Build history of the part. All positions in model axes, mm. Round coordinates to 2 decimals unless told otherwise and drop trailing zeros. Write each loop counter-clockwise with the first axis right and the second up, starting at its lowest first coordinate (ties: lowest second). Pieces come first, ordered by that corner, then holes.
1) Pull direction X, two halves, no side cores. Call faces 1 (the flat face through (0, 6, 5)), 2 (the cylindrical face through (9, -9, 5)), 3 (the flat face through (7, 6, 10)), 4 (the cylindrical face through (6.47, 10.31, 4.93)): +X half, -X half, draft (parallel to the pull), parting line (faces both ways), or undercut.
2) Saw through at D-D (x = 12.5). Write the cut outline in (y, z).
3) Saw through at B-B (x = 8). Write the cut outline in (y, z), plus the area to 3 significant figures.
4) Saw through at C-C (z = 5.5). Write the cut outline in (x, y), plus the area to 3 significant figures.
5) Flat gauge pins, fed straight in: pin 1 (8 mm diameter, centred on x = 9, y = 0, fed in from +Z); pin 2 (4 mm diameter, centred on x = 5, z = 8.5, fed in from +Y). Where does each tip first touch, or does it go through?
6) Saw through at A-A (y = 3.5). Write the cut outline in (x, z), plus the area to 3 significant figures.
7) Wall check: probe 1 along Y at (x, z) = (9, 4.5); probe 2 along Y at (x, z) = (11.25, 3.25); probe 3 along X at (y, z) = (3.5, 6.5). Give the ranges that are in metal, low to high.
from build123d import *

# Parameters (mm, degrees)
SKETCH1_R           = 5
BOSS_EXTRUDE1_DEPTH = 10


with BuildPart() as part:
    # Sketch1 → Boss-Extrude1 (new body)
    with BuildSketch(Plane.XY):
        with BuildLine():
            Line((0, 0), (0, 11.307605315))
            ThreePointArc((0, 11.307605315), (4.336815627, 19.005313513), (13.167713668, 19.284456998))
            ThreePointArc((13.167713668, 19.284456998), (13.418597245, 18.70989145), (12.910980025, 18.341933712))
            ThreePointArc((12.910980025, 18.341933712), (6.518023633, 10.144936613), (16.400138271, 6.919341603))
            ThreePointArc((16.400138271, 6.919341603), (17.447290885, 7.013626461), (18, 6.119237918))
            Line((18, 6.119237918), (18, 0))
            ThreePointArc((18, 0), (9, -9), (0, 0))
        make_face()
        with Locations((9, 0)):
            Circle(SKETCH1_R, mode=Mode.SUBTRACT)
    extrude(amount=BOSS_EXTRUDE1_DEPTH)


solid = part.part
Evaluation:
1. face 1: -X half
1. face 2: parting line
1. face 3: draft
1. face 4: undercut
2. outline: (-8.29, 0) - (-3.57, 0) - (-3.57, 10) - (-8.29, 10) - close; (3.57, 0) - (5.65, 0) - (5.65, 10) - (3.57, 10) - close; (18.35, 0) - (19.6, 0) - (19.6, 10) - (18.35, 10) - close
3. outline: (-8.94, 0) - (-4.9, 0) - (-4.9, 10) - (-8.94, 10) - close; (4.9, 0) - (7.61, 0) - (7.61, 10) - (4.9, 10) - close; (16.39, 0) - (20.25, 0) - (20.25, 10) - (16.39, 10) - close
3. area: 106 mm2
4. outline: (0, 0) arc R9 ccw to (18, 0) - (18, 6.12) arc R1 ccw to (16.4, 6.92) arc R6.35 cw (long way) to (12.91, 18.34) arc R0.5 ccw to (13.17, 19.28) arc R9 ccw to (0, 11.31) - close; hole circle Ø10 at (9, 0)
4. area: 258 mm2
5. pin 1: passes through
5. pin 2: stops at y = 20.08
6. outline: (0, 0) - (5.43, 0) - (5.43, 10) - (0, 10) - close; (12.57, 0) - (18, 0) - (18, 10) - (12.57, 10) - close
6. area: 109 mm2
7. probe 1: y = -9 to -5, 5 to 6.76, 17.24 to 20.31
7. probe 2: y = -8.71 to -4.47, 4.47 to 5.79, 18.21 to 20.02
7. probe 3: x = 0 to 5.43, 12.57 to 18
